Can you work these out from the model? Positions are in its coordinate system, mm. A direction names the side the tool comes from. Coordinates: 2 decimals unless noted, no trailing zeros. Order: outer loops, then holes, each group sorted by start corner. A loop starts at its lowest first (then second) coordinate and runs counter-clockwise, first axis right, second up. Notation, with made-up numbers: M 34,-13.75 L 54,-13.75 A18 ccw 54,-6.75 Z; hole C -36.75,62.25 d11. An arc over 180 degrees is marked long. Answer as a JSON object with one key per item and string values.
from build123d import *

# Parameters (mm, degrees)
F0_R     = 4.4758284469
F1_DEPTH = 25.4


with BuildPart() as f1:
    # F0 (on Front) → F1 (new body)
    with BuildSketch(Plane.XZ):
        with BuildLine():
            ThreePointArc((3.4462378282, 25.9042840516), (0, 24.5743248711), (-3.4462378282, 25.9042840516))
            ThreePointArc((-3.4462378282, 25.9042840516), (0, -26.1325178159), (3.4462378282, 25.9042840516))
        make_face()
        with BuildLine():
            add(Edge.make_bspline(
                [(12.2390337039, -2.3383244956), (10.4852903322, -1.5172076568), (8.7315469605, -1.5172076568)],
                knots=[0, 0, 0, 1, 1, 1], degree=2))
            add(Edge.make_bspline(
                [(8.7315469605, -1.5172076568), (6.1870984848, -1.5172076568), (4.7138188893, -3.2118170998)],
                knots=[0, 0, 0, 1, 1, 1], degree=2))
            add(Edge.make_bspline(
                [(4.7138188893, -3.2118170998), (3.2405392938, -4.9064265428), (3.2405392938, -7.8529857338)],
                knots=[0, 0, 0, 1, 1, 1], degree=2))
            add(Edge.make_bspline(
                [(3.2405392938, -7.8529857338), (3.2405392938, -10.8806428842), (4.6614431238, -12.5347033475)],
                knots=[0, 0, 0, 1, 1, 1], degree=2))
            add(Edge.make_bspline(
                [(4.6614431238, -12.5347033475), (6.0823469539, -14.1887638108), (8.7112724707, -14.1887638108)],
                knots=[0, 0, 0, 1, 1, 1], degree=2))
            add(Edge.make_bspline(
                [(8.7112724707, -14.1887638108), (10.3264734951, -14.1887638108), (12.3978505411, -13.6075617686)],
                knots=[0, 0, 0, 1, 1, 1], degree=2))
            Line((12.3978505411, -13.6075617686), (12.3978505411, -15.1788347317))
            add(Edge.make_bspline(
                [(12.3978505411, -15.1788347317), (10.7927867616, -15.7836903454), (8.4375668577, -15.7836903454)],
                knots=[0, 0, 0, 1, 1, 1], degree=2))
            add(Edge.make_bspline(
                [(8.4375668577, -15.7836903454), (5.0280734819, -15.7836903454), (3.1746472018, -13.7123132994)],
                knots=[0, 0, 0, 1, 1, 1], degree=2))
            add(Edge.make_bspline(
                [(3.1746472018, -13.7123132994), (1.3212209217, -11.6409362535), (1.3212209217, -7.8293321623)],
                knots=[0, 0, 0, 1, 1, 1], degree=2))
            add(Edge.make_bspline(
                [(1.3212209217, -7.8293321623), (1.3212209217, -5.4437005238), (2.2132984749, -3.6494081724)],
                knots=[0, 0, 0, 1, 1, 1], degree=2))
            add(Edge.make_bspline(
                [(2.2132984749, -3.6494081724), (3.1053760281, -1.8551158209), (4.7898482262, -0.8836298491)],
                knots=[0, 0, 0, 1, 1, 1], degree=2))
            add(Edge.make_bspline(
                [(4.7898482262, -0.8836298491), (6.4743204243, 0.0878561227), (8.755200532, 0.0878561227)],
                knots=[0, 0, 0, 1, 1, 1], degree=2))
            add(Edge.make_bspline(
                [(8.755200532, 0.0878561227), (11.1813811503, 0.0878561227), (12.9993270732, -0.7974632673)],
                knots=[0, 0, 0, 1, 1, 1], degree=2))
            Line((12.9993270732, -0.7974632673), (12.2390337039, -2.3383244956))
        make_face(mode=Mode.SUBTRACT)
        Polygon((-6.19505263, 13.6311120435), (-6.19505263, 0), (-7.9617405712, 0), (-7.9617405712, 13.6311120435), (-12.7760483883, 13.6311120435), (-12.7760483883, 15.2015013246), (-1.3807448128, 15.2015013246), (-1.3807448128, 13.6311120435), align=None, mode=Mode.SUBTRACT)
        with BuildLine():
            ThreePointArc((5.1299869915, 29.7043118626), (-2.0781736338, 34.3945102465), (-3.4462378282, 25.9042840516))
            ThreePointArc((-3.4462378282, 25.9042840516), (0, 24.5743248711), (3.4462378282, 25.9042840516))
            ThreePointArc((3.4462378282, 25.9042840516), (4.6901983839, 27.6261382288), (5.1299869915, 29.7043118626))
        make_face()
        with Locations((0, 29.7043118626)):
            Circle(F0_R, mode=Mode.SUBTRACT)
    extrude(amount=F1_DEPTH)


solid = f1.part
Item 1: I want a section at B-B, the plane z = 7.5. Write out the boundary of the cut face in (x, y).
Answers follow:
{"outline": "M -25.03,-25.4 L -7.96,-25.4 L -7.96,0 L -25.03,0 Z; M -6.2,-25.4 L 25.03,-25.4 L 25.03,0 L -6.2,0 Z"}
Item 2: Which directions (+Z, -Z, +X, -X, +Y, -Y) give clear straight access to the entire face, cutting with the end or side of a thin tool? Please do faces 1 (the flat face through (-7.962, -13, 7)), 2 (the flat face through (0, -25.4, -2)).
Answers follow:
{"face 1": "+Y, -Y", "face 2": "+Z, -Z, +X, -X, -Y"}
Item 3: I want a section at C-C, the plane y = -17.75. Give the number of separate pieces and of enclosed holes in the cut face, plus the area to 3 significant figures.
Answers follow:
{"separate pieces": "1", "enclosed holes": "3", "area": "2,060 mm^2"}
Item 4: If we mould it in two halves opening along Z, with no side actions, what happens to faces 3 (the flat face through (0, 0, -2)), 4 (the flat face through (12.398, -13, -14))? For each: pulls with the +Z half, pulls with the -Z half, needs draft (parallel to the pull), parting line crosses it, or undercut.
Answers follow:
{"face 3": "needs draft", "face 4": "undercut"}
Item 5: I want a section at A-A, the plane x = -12. Write out the boundary of the cut face in (y, z), plus the area to 3 significant figures.
Answers follow:
{"outline": "M -25.4,-23.21 L 0,-23.21 L 0,13.63 L -25.4,13.63 Z; M -25.4,15.2 L 0,15.2 L 0,23.21 L -25.4,23.21 Z", "area": "1,140 mm^2"}
Item 6: Please list where these lines run through material, in increasing order: line 1 (X direction, y = -11.5, z = 30); line 2 (Z direction, x = -2.5, y = -13); line 3 (Z direction, x = 10, y = -14.75).
Answers follow:
{"line 1": "x = -5.12 to -4.47, 4.47 to 5.12", "line 2": "z = -26.01 to 13.63, 15.2 to 25.99, 33.42 to 34.18", "line 3": "z = -24.14 to -15.71, -14.11 to -1.62, 0.03 to 24.14"}
Item 7: I'm going to push flat-ended pins straight in: pin 1 (5.5 mm diameter, centred on x = -4.5, y = -12, fed in from +Z); pin 2 (10 mm diameter, centred on y = -15, z = -11, fed in from -X); pin 3 (3 mm diameter, centred on x = 8.5, y = -7.5, fed in from -Z). Where does each tip first touch, or does it pass through?
Answers follow:
{"pin 1": "stops at z = 34.53", "pin 2": "stops at x = -25.43", "pin 3": "stops at z = -25.18"}
Item 8: I want a section at D-D, the plane z = -17.5. Write out the boundary of the cut face in (x, y).
Answers follow:
{"outline": "M -19.41,-25.4 L 19.41,-25.4 L 19.41,0 L -19.41,0 Z"}
